from build123d import *

# Parameters (mm, degrees)
SKETCH1_R           = 4
BOSS_EXTRUDE1_DEPTH = 7


with BuildPart() as part:
    # Sketch1 → Boss-Extrude1 (new body)
    with BuildSketch(Plane.XY.offset(7)):
        with BuildLine():
            Line((16.296858351, 1.939610316), (14.821480939, 2.268299743))
            ThreePointArc((14.821480939, 2.268299743), (14.599363846, 3.384957776), (14.290319486, 4.480746418))
            Line((14.290319486, 4.480746418), (15.455668509, 5.443418171))
            ThreePointArc((15.455668509, 5.443418171), (15.203995461, 6.090594341), (14.924332522, 6.726176719))
            Line((14.924332522, 6.726176719), (13.419594601, 6.582862246))
            ThreePointArc((13.419594601, 6.582862246), (12.863282383, 7.576229188), (12.230746418, 8.522886158))
            Line((12.230746418, 8.522886158), (13.041577269, 9.798554054))
            ThreePointArc((13.041577269, 9.798554054), (12.602233541, 10.336283919), (12.139852525, 10.85433808))
            Line((12.139852525, 10.85433808), (10.753048327, 10.253048327))
            ThreePointArc((10.753048327, 10.253048327), (9.916996701, 11.025886501), (9.022886158, 11.730746418))
            Line((9.022886158, 11.730746418), (9.399829063, 13.194539196))
            ThreePointArc((9.399829063, 13.194539196), (8.815820682, 13.570186009), (8.215982663, 13.920001203))
            Line((8.215982663, 13.920001203), (7.082862246, 12.919594601))
            ThreePointArc((7.082862246, 12.919594601), (6.048909769, 13.396253221), (4.980746418, 13.790319486))
            Line((4.980746418, 13.790319486), (4.88690358, 15.298950909))
            ThreePointArc((4.88690358, 15.298950909), (4.215397354, 15.475743744), (3.536818658, 15.623077622))
            Line((3.536818658, 15.623077622), (2.768299743, 14.321480939))
            ThreePointArc((2.768299743, 14.321480939), (1.637656888, 14.455301339), (0.5, 14.5))
            Line((0.5, 14.5), (-0.055442591, 15.905794714))
            ThreePointArc((-0.055442591, 15.905794714), (-0.748714953, 15.866427856), (-1.439610316, 15.796858351))
            Line((-1.439610316, 15.796858351), (-1.768299743, 14.321480939))
            ThreePointArc((-1.768299743, 14.321480939), (-2.884957776, 14.099363846), (-3.980746418, 13.790319486))
            Line((-3.980746418, 13.790319486), (-4.943418171, 14.955668509))
            ThreePointArc((-4.943418171, 14.955668509), (-5.590594341, 14.703995461), (-6.226176719, 14.424332522))
            Line((-6.226176719, 14.424332522), (-6.082862246, 12.919594601))
            ThreePointArc((-6.082862246, 12.919594601), (-7.076229188, 12.363282383), (-8.022886158, 11.730746418))
            Line((-8.022886158, 11.730746418), (-9.298554054, 12.541577269))
            ThreePointArc((-9.298554054, 12.541577269), (-9.836283919, 12.102233541), (-10.35433808, 11.639852525))
            Line((-10.35433808, 11.639852525), (-9.753048327, 10.253048327))
            ThreePointArc((-9.753048327, 10.253048327), (-10.525886501, 9.416996701), (-11.230746418, 8.522886158))
            Line((-11.230746418, 8.522886158), (-12.694539196, 8.899829063))
            ThreePointArc((-12.694539196, 8.899829063), (-13.070186009, 8.315820682), (-13.420001203, 7.715982663))
            Line((-13.420001203, 7.715982663), (-12.419594601, 6.582862246))
            ThreePointArc((-12.419594601, 6.582862246), (-12.896253221, 5.548909769), (-13.290319486, 4.480746418))
            Line((-13.290319486, 4.480746418), (-14.798950909, 4.38690358))
            ThreePointArc((-14.798950909, 4.38690358), (-14.975743744, 3.715397354), (-15.123077622, 3.036818658))
            Line((-15.123077622, 3.036818658), (-13.821480939, 2.268299743))
            ThreePointArc((-13.821480939, 2.268299743), (-13.955301339, 1.137656888), (-14, 0))
            Line((-14, 0), (-15.405794714, -0.555442591))
            ThreePointArc((-15.405794714, -0.555442591), (-15.366427856, -1.248714953), (-15.296858351, -1.939610316))
            Line((-15.296858351, -1.939610316), (-13.821480939, -2.268299743))
            ThreePointArc((-13.821480939, -2.268299743), (-13.599363846, -3.384957776), (-13.290319486, -4.480746418))
            Line((-13.290319486, -4.480746418), (-14.455668509, -5.443418171))
            ThreePointArc((-14.455668509, -5.443418171), (-14.203995461, -6.090594341), (-13.924332522, -6.726176719))
            Line((-13.924332522, -6.726176719), (-12.419594601, -6.582862246))
            ThreePointArc((-12.419594601, -6.582862246), (-11.863282383, -7.576229188), (-11.230746418, -8.522886158))
            Line((-11.230746418, -8.522886158), (-12.041577269, -9.798554054))
            ThreePointArc((-12.041577269, -9.798554054), (-11.602233541, -10.336283919), (-11.139852525, -10.85433808))
            Line((-11.139852525, -10.85433808), (-9.753048327, -10.253048327))
            ThreePointArc((-9.753048327, -10.253048327), (-8.916996701, -11.025886501), (-8.022886158, -11.730746418))
            Line((-8.022886158, -11.730746418), (-8.399829063, -13.194539196))
            ThreePointArc((-8.399829063, -13.194539196), (-7.815820682, -13.570186009), (-7.215982663, -13.920001203))
            Line((-7.215982663, -13.920001203), (-6.082862246, -12.919594601))
            ThreePointArc((-6.082862246, -12.919594601), (-5.048909769, -13.396253221), (-3.980746418, -13.790319486))
            Line((-3.980746418, -13.790319486), (-3.88690358, -15.298950909))
            ThreePointArc((-3.88690358, -15.298950909), (-3.215397354, -15.475743744), (-2.536818658, -15.623077622))
            Line((-2.536818658, -15.623077622), (-1.768299743, -14.321480939))
            ThreePointArc((-1.768299743, -14.321480939), (-0.637656888, -14.455301339), (0.5, -14.5))
            Line((0.5, -14.5), (1.055442591, -15.905794714))
            ThreePointArc((1.055442591, -15.905794714), (1.748714953, -15.866427856), (2.439610316, -15.796858351))
            Line((2.439610316, -15.796858351), (2.768299743, -14.321480939))
            ThreePointArc((2.768299743, -14.321480939), (3.884957776, -14.099363846), (4.980746418, -13.790319486))
            Line((4.980746418, -13.790319486), (5.943418171, -14.955668509))
            ThreePointArc((5.943418171, -14.955668509), (6.590594341, -14.703995461), (7.226176719, -14.424332522))
            Line((7.226176719, -14.424332522), (7.082862246, -12.919594601))
            ThreePointArc((7.082862246, -12.919594601), (8.076229188, -12.363282383), (9.022886158, -11.730746418))
            Line((9.022886158, -11.730746418), (10.298554054, -12.541577269))
            ThreePointArc((10.298554054, -12.541577269), (10.836283919, -12.102233541), (11.35433808, -11.639852525))
            Line((11.35433808, -11.639852525), (10.753048327, -10.253048327))
            ThreePointArc((10.753048327, -10.253048327), (11.525886501, -9.416996701), (12.230746418, -8.522886158))
            Line((12.230746418, -8.522886158), (13.694539196, -8.899829063))
            ThreePointArc((13.694539196, -8.899829063), (14.070186009, -8.315820682), (14.420001203, -7.715982663))
            Line((14.420001203, -7.715982663), (13.419594601, -6.582862246))
            ThreePointArc((13.419594601, -6.582862246), (13.896253221, -5.548909769), (14.290319486, -4.480746418))
            Line((14.290319486, -4.480746418), (15.798950909, -4.38690358))
            ThreePointArc((15.798950909, -4.38690358), (15.975743744, -3.715397354), (16.123077622, -3.036818658))
            Line((16.123077622, -3.036818658), (14.821480939, -2.268299743))
            ThreePointArc((14.821480939, -2.268299743), (14.955301339, -1.137656888), (15, 0))
            Line((15, 0), (16.405794714, 0.555442591))
            ThreePointArc((16.405794714, 0.555442591), (16.366427856, 1.248714953), (16.296858351, 1.939610316))
        make_face()
        with Locations((0.5, 0)):
            Circle(SKETCH1_R, mode=Mode.SUBTRACT)
    extrude(amount=-BOSS_EXTRUDE1_DEPTH)


solid = part.part
Verification items for the finished model (mm, model axes). A direction names the side the tool comes from. Coordinates: 2 decimals unless noted, no trailing zeros. Order: outer loops, then holes, each group sorted by start corner. A loop starts at its lowest first (then second) coordinate and runs counter-clockwise, first axis right, second up. Notation, with made-up numbers: M -22.75,47 L 18.25,47 A19 ccw 18.25,81 Z; hole C 7,63 d8. An arc over 180 degrees is marked long. One line per item, written item: value. Start each with the question number.
Item 1: Access from +Z, -Z, +X, -X, +Y, -Y to the whole of each face (thin tool, end or side, straight path). Record for faces 1 (the flat face through (-2.158, -14.981, 3.549)), 2 (the cylindrical face through (11.516, -9.429, 3.549)), 3 (the flat face through (-6.156, 13.682, 3.549)), 4 (the flat face through (14.182, 6.656, 3.549)).
Item 2: Depth check by flat-ended pin: P1, Ø4, axis at x = 7.5, z = 2, coming from the -Y side; P2, Ø3, axis at x = -4.5, z = 4, coming from the +Y side; P3, Ø3, axis at y = -4, z = 2.5, coming from the +X side. Enter the tip coordinate at first touch or a pass-through.
Item 3: Mould release check, pull along X, two halves, no side actions. Record for faces 5 (the flat face through (11.06, -10.96, 3.55)), 6 (the cylindrical face through (-0.367, -3.905, 3.549)), 7 (the flat face through (-12.93, 7.16, 3.55)), 8 (the flat face through (5.455, -14.365, 3.549)): pulls with the +X half, pulls with the -X half, needs draft (parallel to the pull), parting line crosses it, or undercut.
Item 4: Sectioned sample at A-A on x = -5.5. Record the cut outline in (y, z), then the cut area to 3 significant figures.
Item 5: Thickness scan on probe 1 along X at (y, z) = (-5.5, 3.5); probe 2 along X at (y, z) = (-12, 2); probe 3 along Y at (x, z) = (13.5, 6). Record the ranges inside material, lowest first.
Calculated:
1. face 1: +Z, -Z, -Y
1. face 2: +Z, -Z
1. face 3: +Z, -Z, -X
1. face 4: +Z, -Z, +Y
2. P1: y = -14.96
2. P2: y = 14.96
2. P3: x = 16.12
3. face 5: pulls with the +X half
3. face 6: undercut
3. face 7: pulls with the -X half
3. face 8: undercut
4. outline: M -13.2,0 L 14.74,0 L 14.74,7 L -13.2,7 Z
4. area: 196 mm^2
5. probe 1: -14.43 to 13.92
5. probe 2: -8.09 to 8.64, 9.45 to 10.95
5. probe 3: -8.85 to -6.67, -6.42 to 6.59
